Autodesk Inventor part; units mm, degrees
ref_plane "Work Plane1" through (0, 0, 10) normal (0, 0, 1) x (1, 0, 0)
ref_plane "Work Plane4" through (-20.9299, 20.9299, 36.9) normal (-1, 0, 0) x (0, 1, 0)
ref_plane "YZ Plane" through (0, 0, 0) normal (1, 0, 0) x (0, 1, 0)
ref_plane "Work Plane1" through (0, 0, 10) normal (0, 0, 1) x (1, 0, 0)
sketch "Sketch1" plane through (0, 0, 10) normal (0, 0, 1) x (1, 0, 0)
  line L0 (-4.0299, -0.3538) -> (-2.2322, 1.4439) construction
  arc A0 (-1.4439, 2.2322) -> (-2.2322, 1.4439) centre (-0.9299, 0.9299) ccw construction
  line L1 (-1.4439, 2.2322) -> (0.3538, 4.0299) construction
  line L2 (-37.8299, 42.2137) -> (-37.8299, 45.8299) construction
  line L3 (-37.8299, 45.8299) -> (-4.0299, 45.8299) construction
  line L4 (-4.0299, 45.8299) -> (-4.0299, 42.2137) construction
  line L5 (-4.0299, 4.0299) -> (0.3538, 4.0299)
  circle A1 centre (-20.9299, 20.9299) radius 17.5
  line L6 (-20.9299, 58.9723) -> (17.1124, 20.9299) construction
  line L7 (17.1124, 20.9299) -> (-20.9299, -17.1124) construction
  line L8 (-20.9299, -17.1124) -> (-58.9723, 20.9299) construction
  line L9 (-58.9723, 20.9299) -> (-20.9299, 58.9723) construction
  line L10 (-20.9299, 58.9723) -> (-20.9299, -17.1124) construction
  line L11 (17.1124, 20.9299) -> (-58.9723, 20.9299) construction
  line L12 (-20.9299, 58.9723) -> (32.8701, 58.9723) construction
  line L13 (-43.4299, 43.4299) -> (1.5701, 43.4299) construction
  line L14 (1.5701, 43.4299) -> (1.5701, -1.5701) construction
  line L15 (1.5701, -1.5701) -> (-43.4299, -1.5701) construction
  line L16 (-43.4299, -1.5701) -> (-43.4299, 43.4299) construction
  line L17 (-43.4299, 43.4299) -> (1.5701, -1.5701) construction
  line L18 (1.5701, 43.4299) -> (-43.4299, -1.5701) construction
  line L19 (-43.4299, 5.3876) -> (-43.4299, 36.4723)
  line L20 (-43.4299, 36.4723) -> (-36.4723, 43.4299)
  line L21 (-36.4723, 43.4299) -> (-5.3876, 43.4299)
  line L22 (-5.3876, 43.4299) -> (1.5701, 36.4723)
  line L23 (1.5701, 36.4723) -> (1.5701, 5.3876)
  line L24 (1.5701, 5.3876) -> (-5.3876, -1.5701)
  line L25 (-5.3876, -1.5701) -> (-36.4723, -1.5701)
  line L26 (-36.4723, -1.5701) -> (-43.4299, 5.3876)
  line L27 (-4.0299, 42.2137) -> (-37.8299, 42.2137)
  line L28 (-4.0299, -0.3538) -> (-4.0299, 4.0299)
  circle A2 centre (-20.9299, 20.9299) radius 7.0417
  point P0 (-37.8299, 4.0299)
  dimension "d18" = 53.8
  dimension "d19" = 45
  dimension "d20" = 53.8
  dimension "d21" = 45
  dimension "d22" = 45
extrude "Extrusion1" add sketch "Sketch1" along normal blind 3 contours L28 L24 L25 L26 L19 L20 L27 L22 L23 L5 | L5 L24 L28 | L27 L20 L21 L22 | A1
sketch "Sketch3" plane through (0, 0, 10) normal (0, 0, -1) x (-1, 0, 0)
  line L0 (37.8299, -0.4701) -> (37.8299, 4.0299) construction
  line L1 (4.0299, 4.0299) -> (4.0299, -0.4701) construction
  line L2 (37.8299, -0.4701) -> (37.8299, 1.1886) construction
  line L3 (4.0299, -3.9701) -> (4.0299, -0.3538) construction
  line L4 (45.8299, 4.0299) -> (42.2137, 4.0299) construction
  line L5 (-0.3538, 4.0299) -> (-3.9701, 4.0299) construction
  line L6 (-3.9701, 37.8299) -> (-0.3538, 37.8299) construction
  line L7 (4.0299, 42.2137) -> (4.0299, 45.8299) construction
  line L8 (37.8299, 45.8299) -> (37.8299, 42.2137) construction
  line L9 (42.2137, 37.8299) -> (45.8299, 37.8299) construction
  line L10 (37.8299, 37.7299) -> (45.8299, 37.7299)
  line L11 (45.8299, 37.7299) -> (45.8299, 4.1299)
  line L12 (45.8299, 4.1299) -> (37.8299, 4.1299)
  line L13 (37.8299, 4.1299) -> (37.8299, 37.7299)
  line L14 (37.7299, 4.0299) -> (4.1299, 4.0299)
  line L15 (4.1299, 4.0299) -> (4.1299, -3.9701)
  line L16 (4.1299, -3.9701) -> (37.7299, -3.9701)
  line L17 (37.7299, -3.9701) -> (37.7299, 4.0299)
  line L18 (4.0299, 4.1299) -> (-3.9701, 4.1299)
  line L19 (-3.9701, 4.1299) -> (-3.9701, 37.7299)
  line L20 (-3.9701, 37.7299) -> (4.0299, 37.7299)
  line L21 (4.0299, 37.7299) -> (4.0299, 4.1299)
  line L22 (4.1299, 37.8299) -> (37.7299, 37.8299)
  line L23 (37.7299, 37.8299) -> (37.7299, 45.8299)
  line L24 (37.7299, 45.8299) -> (4.1299, 45.8299)
  line L25 (4.1299, 45.8299) -> (4.1299, 37.8299)
  point P0 (0, 0)
  dimension "d23" = 0.1
  dimension "d24" = 0.1
  dimension "d25" = 0.1
  dimension "d26" = 0.1
  dimension "d27" = 0.1
extrude "Extrusion3" add sketch "Sketch3" against normal up to surface (3 mm away)
ref_plane "Work Plane4" through (-20.9299, 20.9299, 36.9) normal (-1, 0, 0) x (0, 1, 0)
sketch "Sketch11" plane through (-20.9299, 20.9299, 36.9) normal (-1, 0, 0) x (0, 1, 0)
  point P0 (-20.9299, 36.9)
sketch "Sketch12" plane through (0, 0, 13) normal (0, 0, 1) x (1, 0, 0)
  line L0 (-11.9799, 39.5299) -> (-11.9799, 43.8299) construction
  line L1 (-17.0799, -2.9701) -> (-17.0799, 2.0299) construction
  line L2 (-37.7299, 45.8299) -> (-4.1299, 45.8299)
  line L3 (-20.9299, 45.8299) -> (-20.9299, -3.9701)
  line L4 (-4.1299, -3.9701) -> (-37.7299, -3.9701)
  line L5 (-20.9299, -3.9701) -> (-15.0511, -3.9701)
  line L6 (-15.0511, -3.9701) -> (-15.0511, 9.6316)
  line L7 (-20.9299, 45.8299) -> (-9.9943, 45.8299)
  line L8 (-9.9943, 45.8299) -> (-9.9943, 35.0551)
  line L9 (-9.9943, 35.0551) -> (-12.2675, 24.6166) construction
  line L10 (-12.2675, 24.6166) -> (-15.0511, 18.1216) construction
  line L11 (-15.0511, 18.1216) -> (-15.0511, 9.6316) construction
  spline S0 degree 3 poles (-9.9943, 35.0551) (-12.2675, 24.6166) (-15.0511, 18.1216) (-15.0511, 9.6316) knots 1 1 1 1 2 2 2 2
  point P0 (0, 0)
extrude "Extrusion10" add sketch "Sketch12" along normal blind 15
sketch "Sketch13" plane through (-20.9299, 13.8882, 13) normal (-1, 0, 0) x (0, 0, 1)
  line L0 (34.8, 31.9417) -> (-5, 31.9417)
  line L1 (36.8, -17.8583) -> (-5, -17.8583) construction
  line L2 (0, -17.8583) -> (15, -17.8583)
  line L3 (11.9179, -17.8583) -> (11.9179, 31.9417)
  line L4 (-5, 29.9417) -> (34.8, 29.9417) construction
  line L5 (16, -16.8583) -> (16, -11.8583) construction
  line L6 (9.0528, -16.8583) -> (9.0528, -11.8583) construction
  line L7 (9.709, -7.8145) -> (9.709, -17.8583)
  line L8 (9.709, -17.8583) -> (11.9179, -17.8583)
  arc A0 (5.7696, 30.9102) -> (2.95, 29.9417) centre (11.845, 8.6329) ccw
  line L9 (11.9179, 31.9417) -> (7.5, 31.9417)
  line L10 (0, 31.9417) -> (15, 31.9417)
  line L11 (9.709, -17.8583) -> (11.9179, -17.8583)
  line L12 (2.95, 29.9417) -> (2.95, 25.6417)
  line L13 (2.95, 25.6417) -> (4.6268, 25.6417)
  line L14 (7.5, 31.9417) -> (5.7696, 31.9417)
  line L15 (5.7696, 30.9102) -> (5.7696, 31.9417)
  line L16 (4.6268, 25.6417) -> (4.6268, 11.6155) construction
  line L17 (0, 21.1669) -> (15, 21.1669)
  line L18 (4.6268, 11.6155) -> (5.7696, 2.2174) construction
  line L19 (5.7696, 2.2174) -> (9.709, 3.7875) construction
  line L20 (9.709, 3.7875) -> (9.709, -7.8145) construction
  spline S0 degree 4 poles (4.6268, 25.6417) (4.6268, 11.6155) (5.7696, 2.2174) (9.709, 3.7875) (9.709, -7.8145) knots 1 1 1 1 1 2 2 2 2 2
  point P0 (-13, -13.8882)
  dimension "d69" = 4.4179
revolve "Revolution1" cut sketch "Sketch13" angle 360 about axis through (-20.9299, -3.9701, 24.9179) along (0, 1, 0)
sketch "Sketch14" plane through (-37.7299, -3.9701, 10) normal (0, -1, 0) x (1, 0, 0)
  circle A0 centre (16.8, 14.9) radius 2.8472
  line L0 (12.95, 19) -> (20.65, 19)
  line L1 (12.95, 10.8) -> (12.95, 19)
  line L2 (20.65, 10.8) -> (12.95, 10.8)
  line L3 (20.65, 19) -> (20.65, 10.8)
  line L4 (20.85, 19.2) -> (12.75, 19.2)
  line L5 (12.75, 19.2) -> (12.75, 10.6)
  line L6 (12.75, 10.6) -> (20.85, 10.6)
  line L7 (20.85, 10.6) -> (20.85, 19.2)
  point P0 (37.7299, -10)
  dimension "d66" = 0.2
extrude "Extrusion11" cut sketch "Sketch14" against normal through all contours A0 | L0 L3 L2 L1 | L7 L6 L5 L4
mirror "Mirror1" about plane through (-20.9299, 45.8299, 13) normal (-1, 0, 0) of "Extrusion10", "Revolution1", "Extrusion11"
properties part number "20_Cube_Insert_Beamexpander"
Geometry check sheet. Reference: the model listing, model coordinates, mm. A direction names the side the tool comes from. Coordinates: 2 decimals unless noted, no trailing zeros. Order: outer loops, then holes, each group sorted by start corner. A loop starts at its lowest first (then second) coordinate and runs counter-clockwise, first axis right, second up.
Q1. Sectioned sample at A-A on y = 41. Record the cut outline in (x, z), and give its area (3 significant figures).
Reply:
outline: (-38.9, 10) - (-2.96, 10) - (-2.96, 13) - (-9.99, 13) - (-9.99, 28) - (-12.51, 28) arc R8.97 cw (long way) to (-29.35, 28) - (-31.87, 28) - (-31.87, 13) - (-38.9, 13) - close
area: 255 mm2
Q2. Sectioned sample at B-B on x = -6. Record the cut outline in (y, z).
Reply:
outline: (-3.97, 10) - (45.83, 10) - (45.83, 13) - (-3.97, 13) - close
Q3. Depth check by flat-ended pin: pin 1 Ø3.5 at (y, z) = (-2, 12) entering from +X; pin 2 Ø10 at (x, z) = (-37, 19.5) entering from +Y; pin 3 Ø4 at (x, y) = (-20.5, 7.5) entering from +Z; pin 4 Ø2 at (y, z) = (6.5, 24) entering from +X. Enter the tip coordinate at first touch or a pass-through.
Reply:
pin 1: stops at x = -4.07
pin 2: passes through
pin 3: stops at z = 20.6
pin 4: stops at x = -15.05
Q4. Thickness scan on probe 1 along X at (y, z) = (4, 22.5); probe 2 along Z at (x, y) = (-5, 12); probe 3 along X at (y, z) = (16, 20.75). Record the ranges inside material, lowest first.
Reply:
probe 1: x = -26.81 to -24.98, -16.88 to -15.05
probe 2: z = 10 to 13
probe 3: x = -27.32 to -24.98, -16.88 to -14.54
Q5. Draft check along X on faces 1 (the face through (-40, 39.9, 11.5)), 2 (the face through (-21, 45.83, 17)), 3 (the face through (-24.98, 6, 24)), 4 (the face through (-15.051, 3, 20)). Enter one of: released by +X, released by -X, zero draft, split by the parting line, or undercut.
Reply:
face 1: released by -X
face 2: zero draft
face 3: undercut
face 4: released by +X
Q6. Sectioned sample at C-C on y = 1.5. Record the cut outline in (x, z).
Reply:
outline: (-39.54, 10) - (-2.32, 10) - (-2.32, 13) - (-15.05, 13) - (-15.05, 28) - (-16.88, 28) - (-16.88, 20.6) - (-24.98, 20.6) - (-24.98, 28) - (-26.81, 28) - (-26.81, 13) - (-39.54, 13) - close
Q7. Tool access check on faces 5 (the face through (-31.866, 40, 20)), 6 (the face through (-22.3, 39.53, 17.5)), 7 (the face through (-37.73, 44, 11)), 8 (the face through (-44, 4.13, 11)). Record the directions out of +Z, -Z, +X, -X, +Y, -Y that give a thin tool (end or side, any length) a straight path to the whole face; none if there is none.
Reply:
face 5: +Z, -X, +Y, -Y
face 6: none
face 7: +Z, -Z, -X, +Y
face 8: +Z, -Z, -X, -Y
